from build123d import *

# Parameters (mm, degrees)
SKETCH_1_W          = 275.5
SKETCH_1_H          = 88.9
EXTRUDE_1_DEPTH     = 10
FILLET_1_R          = 10
CUT_EXTRUDE_1_DEPTH = 10
CHAMFER_2_SIZE      = 2
FILLET_3_R          = 3
SKETCH_3_W          = 255.5
SKETCH_3_H          = 3
CUT_EXTRUDE_2_DEPTH = 4
SKETCH_4_R          = 1.5
CUT_EXTRUDE_3_DEPTH = 46
CUT_EXTRUDE_START   = -4
SKETCH_5_R          = 3
SKETCH_5_R_2        = 1.5
CUT_EXTRUDE_4_DEPTH = 4
SKETCH_6_W          = 135.5
SKETCH_6_H          = 3
EXTRUDE_2_DEPTH     = 3


with BuildPart() as part:
    # 草图1 → 凸台-拉伸1 (new body)
    with BuildSketch(Plane.XY):
        Rectangle(SKETCH_1_W, SKETCH_1_H)
    extrude(amount=EXTRUDE_1_DEPTH)

    # 圆角1
    fillet_1_edges = [part.edges().sort_by_distance(p)[0] for p in [
        (137.75, -44.45, 5),
        (-137.75, -44.45, 5),
        (-137.75, 44.45, 5),
        (137.75, 44.45, 5),
    ]]
    fillet(fillet_1_edges, radius=FILLET_1_R)

    # 草图2 → 切除-拉伸1 (cut)
    with BuildSketch(Plane.XY.offset(10)):
        with BuildLine():
            Line((-6.25, 30.95), (6.25, 30.95))
            ThreePointArc((6.25, 30.95), (13.321067812, 28.021067812), (16.25, 20.95))
            Line((16.25, 20.95), (16.25, -20.95))
            ThreePointArc((16.25, -20.95), (13.321067812, -28.021067812), (6.25, -30.95))
            Line((6.25, -30.95), (-6.25, -30.95))
            ThreePointArc((-6.25, -30.95), (-13.787950414, -27.521096069), (-16.156519268, -19.58586071))
            Line((-16.156519268, -19.58586071), (-16.156519268, 19.58586071))
            ThreePointArc((-16.156519268, 19.58586071), (-13.787950414, 27.521096069), (-6.25, 30.95))
        make_face()
        with BuildLine():
            Line((-43.75, -30.95), (-56.25, -30.95))
            ThreePointArc((-56.25, -30.95), (-63.787950414, -27.521096069), (-66.156519268, -19.58586071))
            Line((-66.156519268, -19.58586071), (-66.156519268, 19.58586071))
            ThreePointArc((-66.156519268, 19.58586071), (-63.787950414, 27.521096069), (-56.25, 30.95))
            Line((-56.25, 30.95), (-43.75, 30.95))
            ThreePointArc((-43.75, 30.95), (-36.678932188, 28.021067812), (-33.75, 20.95))
            Line((-33.75, 20.95), (-33.75, -20.95))
            ThreePointArc((-33.75, -20.95), (-36.678932188, -28.021067812), (-43.75, -30.95))
        make_face()
        with BuildLine():
            Line((56.25, -30.95), (43.75, -30.95))
            ThreePointArc((43.75, -30.95), (36.212049586, -27.521096069), (33.843480732, -19.58586071))
            Line((33.843480732, -19.58586071), (33.843480732, 19.58586071))
            ThreePointArc((33.843480732, 19.58586071), (36.212049586, 27.521096069), (43.75, 30.95))
            Line((43.75, 30.95), (56.25, 30.95))
            ThreePointArc((56.25, 30.95), (63.321067812, 28.021067812), (66.25, 20.95))
            Line((66.25, 20.95), (66.25, -20.95))
            ThreePointArc((66.25, -20.95), (63.321067812, -28.021067812), (56.25, -30.95))
        make_face()
        with BuildLine():
            Line((106.25, -30.95), (93.75, -30.95))
            ThreePointArc((93.75, -30.95), (86.212049586, -27.521096069), (83.843480732, -19.58586071))
            Line((83.843480732, -19.58586071), (83.843480732, 19.58586071))
            ThreePointArc((83.843480732, 19.58586071), (86.212049586, 27.521096069), (93.75, 30.95))
            Line((93.75, 30.95), (106.25, 30.95))
            ThreePointArc((106.25, 30.95), (113.321067812, 28.021067812), (116.25, 20.95))
            Line((116.25, 20.95), (116.25, -20.95))
            ThreePointArc((116.25, -20.95), (113.321067812, -28.021067812), (106.25, -30.95))
        make_face()
        with BuildLine():
            Line((-93.75, -30.95), (-106.25, -30.95))
            ThreePointArc((-106.25, -30.95), (-113.787950414, -27.521096069), (-116.156519268, -19.58586071))
            Line((-116.156519268, -19.58586071), (-116.156519268, 19.58586071))
            ThreePointArc((-116.156519268, 19.58586071), (-113.787950414, 27.521096069), (-106.25, 30.95))
            Line((-106.25, 30.95), (-93.75, 30.95))
            ThreePointArc((-93.75, 30.95), (-86.678932188, 28.021067812), (-83.75, 20.95))
            Line((-83.75, 20.95), (-83.75, -20.95))
            ThreePointArc((-83.75, -20.95), (-86.678932188, -28.021067812), (-93.75, -30.95))
        make_face()
    extrude(amount=-CUT_EXTRUDE_1_DEPTH, mode=Mode.SUBTRACT)

    # 倒角2
    chamfer_2_edges = [part.edges().sort_by_distance(p)[0] for p in [
        (86.212049586, 27.521096069, 10),
        (83.843480732, 0, 10),
        (86.212049586, -27.521096069, 10),
        (100, -30.95, 10),
        (113.321067812, -28.021067812, 10),
        (116.25, 0, 10),
        (113.321067812, 28.021067812, 10),
        (100, 30.95, 10),
        (-113.787950414, 27.521096069, 10),
        (-116.156519268, 0, 10),
        (-113.787950414, -27.521096069, 10),
        (-100, -30.95, 10),
        (-86.678932188, -28.021067812, 10),
        (-83.75, 0, 10),
        (-86.678932188, 28.021067812, 10),
        (-100, 30.95, 10),
        (-13.787950414, 27.521096069, 10),
        (-16.156519268, 0, 10),
        (-13.787950414, -27.521096069, 10),
        (0, -30.95, 10),
        (13.321067812, -28.021067812, 10),
        (16.25, 0, 10),
        (13.321067812, 28.021067812, 10),
        (0, 30.95, 10),
        (36.212049586, 27.521096069, 10),
        (33.843480732, 0, 10),
        (36.212049586, -27.521096069, 10),
        (50, -30.95, 10),
        (63.321067812, -28.021067812, 10),
        (66.25, 0, 10),
        (63.321067812, 28.021067812, 10),
        (50, 30.95, 10),
        (-63.787950414, 27.521096069, 10),
        (-66.156519268, 0, 10),
        (-63.787950414, -27.521096069, 10),
        (-50, -30.95, 10),
        (-36.678932188, -28.021067812, 10),
        (-33.75, 0, 10),
        (-36.678932188, 28.021067812, 10),
        (-50, 30.95, 10),
    ]]
    chamfer(chamfer_2_edges, length=CHAMFER_2_SIZE)

    # 圆角3
    fillet_3_edges = [part.edges().sort_by_distance(p)[0] for p in [
        (0, -44.45, 10),
        (-137.75, 0, 10),
        (137.75, 0, 10),
        (0, 44.45, 10),
        (-134.821067812, 41.521067812, 10),
        (134.821067812, 41.521067812, 10),
        (134.821067812, -41.521067812, 10),
        (-134.821067812, -41.521067812, 10),
    ]]
    fillet(fillet_3_edges, radius=FILLET_3_R)

    # 草图3 → 切除-拉伸2 (cut)
    with BuildSketch(Plane(origin=(0, 0, 0), x_dir=(-1, 0, 0), z_dir=(0, 0, -1))):
        with Locations((0, -40.45)):
            Rectangle(SKETCH_3_W, SKETCH_3_H)
    extrude(amount=-CUT_EXTRUDE_2_DEPTH, mode=Mode.SUBTRACT)

    # 草图4 → 切除-拉伸3 (cut)
    with BuildSketch(Plane(origin=(0, 0, 0), x_dir=(-1, 0, 0), z_dir=(0, 0, -1))):
        with Locations((-130.75, 37.45)):
            Circle(SKETCH_4_R)
        with Locations((130.75, 37.45)):
            Circle(SKETCH_4_R)
        with Locations((130.75, -37.45)):
            Circle(SKETCH_4_R)
        with Locations((-130.75, -37.45)):
            Circle(SKETCH_4_R)
        with Locations((67.75, 37.45)):
            Circle(SKETCH_4_R)
        with Locations((-130.75, 0)):
            Circle(SKETCH_4_R)
        with Locations((130.75, 0)):
            Circle(SKETCH_4_R)
    extrude(amount=-CUT_EXTRUDE_3_DEPTH, mode=Mode.SUBTRACT)

    # 草图5 → 切除-拉伸4 (cut)
    # profile 1 of 7: a face of its own
    with BuildSketch(Plane.XY.offset(10).offset(CUT_EXTRUDE_START)):
        with Locations((-67.75, 37.45)):
            Circle(SKETCH_5_R)
        with Locations(Location((-67.75, 37.45, 0), (0, 0, 180))):
            Circle(SKETCH_5_R_2, mode=Mode.SUBTRACT)
    # profile 2 of 7: a face of its own
    with BuildSketch(Plane.XY.offset(10).offset(CUT_EXTRUDE_START)):
        with Locations((130.75, 0)):
            Circle(SKETCH_5_R)
        with Locations(Location((130.75, 0, 0), (0, 0, 180))):
            Circle(SKETCH_5_R_2, mode=Mode.SUBTRACT)
    # profile 3 of 7: a face of its own
    with BuildSketch(Plane.XY.offset(10).offset(CUT_EXTRUDE_START)):
        with Locations((-130.75, 0)):
            Circle(SKETCH_5_R)
        with Locations(Location((-130.75, 0, 0), (0, 0, 180))):
            Circle(SKETCH_5_R_2, mode=Mode.SUBTRACT)
    # profile 4 of 7: a face of its own
    with BuildSketch(Plane.XY.offset(10).offset(CUT_EXTRUDE_START)):
        with Locations((-130.75, 37.45)):
            Circle(SKETCH_5_R)
        with Locations(Location((-130.75, 37.45, 0), (0, 0, 180))):
            Circle(SKETCH_5_R_2, mode=Mode.SUBTRACT)
    # profile 5 of 7: a face of its own
    with BuildSketch(Plane.XY.offset(10).offset(CUT_EXTRUDE_START)):
        with Locations((-130.75, -37.45)):
            Circle(SKETCH_5_R)
        with Locations(Location((-130.75, -37.45, 0), (0, 0, 180))):
            Circle(SKETCH_5_R_2, mode=Mode.SUBTRACT)
    # profile 6 of 7: a face of its own
    with BuildSketch(Plane.XY.offset(10).offset(CUT_EXTRUDE_START)):
        with Locations((130.75, 37.45)):
            Circle(SKETCH_5_R)
        with Locations(Location((130.75, 37.45, 0), (0, 0, 180))):
            Circle(SKETCH_5_R_2, mode=Mode.SUBTRACT)
    # profile 7 of 7: a face of its own
    with BuildSketch(Plane.XY.offset(10).offset(CUT_EXTRUDE_START)):
        with Locations((130.75, -37.45)):
            Circle(SKETCH_5_R)
        with Locations(Location((130.75, -37.45, 0), (0, 0, 180))):
            Circle(SKETCH_5_R_2, mode=Mode.SUBTRACT)
    extrude(amount=CUT_EXTRUDE_4_DEPTH, mode=Mode.SUBTRACT)

    # 草图6 → 凸台-拉伸2 (add)
    with BuildSketch(Plane(origin=(0, 0, 0), x_dir=(-1, 0, 0), z_dir=(0, 0, -1))):
        with Locations((-10, 39.45)):
            Rectangle(SKETCH_6_W, SKETCH_6_H)
    extrude(amount=EXTRUDE_2_DEPTH)


solid = part.part
Geometry check sheet. Reference: the model listing, model coordinates, mm. A direction names the side the tool comes from. Round coordinates to 2 decimals unless told otherwise and drop trailing zeros. Order: outer loops, then holes, each group sorted by start corner. A loop starts at its lowest first (then second) coordinate and runs counter-clockwise, first axis right, second up. Notation, with made-up numbers: M 44,18 L 91,18 A33 ccw 91,46 Z; hole C 71.5,-28 d2. An arc over 180 degrees is marked long. Write each question's results on one line, items separated by ' | '. Start each with the question number.
1. Material ranges on L1, parallel to Y at x = 1.5, z = 2.25; L2, parallel to X at y = -4, z = 2.75; L3, parallel to Y at x = 130.75, z = 4.7, recorded low to high. Write a range as from..to.
2. Cross-section at A-A on x = -51. Record the boundary of the cut face in (y, z), plus the area to 3 significant figures.
3. Draft check along Y on faces 1 (the face through (13.786, -28.322, 8.542)), 2 (the face through (86.05, -27.82, 8.32)), 3 (the face through (134.74, -41.6, 3.55)). Enter one of: pulls with the +Y half, pulls with the -Y half, needs draft (parallel to the pull), parting line crosses it, or undercut.
4. Set-up check for faces 4 (the face through (-113.95, -27.82, 8.32)), 5 (the face through (-50, 30.95, 4)), 6 (the face through (-2, -44.45, 3)): record each of +Z, -Z, +X, -X, +Y, -Y from which the full face is reachable in a straight line by a thin tool's end or side.
5. Go/stop test with flat-tipped pins: P1, Ø1, axis at x = 98.5, y = -30.5, coming from the +Z side; P2, Ø1.5, axis at x = 18, y = 34, coming from the -Z side; P3, Ø1.8, axis at x = 131, y = -0.5, coming from the +Z side. Record where each tip stops, or that it passes through.
6. Cross-section at B-B on y = 11. Give the number of separate pieces and of enclosed holes in the cut face, plus the area to 3 significant figures.
Resolved:
1) L1: -44.45..-41.95, -38.95..-30.95, 30.95..44.45 | L2: -137.75..-116.16, -83.75..-66.16, -33.75..-16.16, 16.25..33.84, 66.25..83.84, 116.25..137.75 | L3: -43.99..-38.95, -35.95..-1.5, 1.5..35.95, 38.95..43.99
2) outline: M -44.45,0 L -41.95,0 L -41.95,4 L -38.95,4 L -38.95,0 L -30.95,0 L -30.95,8 L -32.95,10 L -41.45,10 A3 ccw -44.45,7 Z; M 30.95,0 L 37.95,0 L 37.95,-3 L 40.95,-3 L 40.95,0 L 44.45,0 L 44.45,7 A3 ccw 41.45,10 L 32.95,10 L 30.95,8 Z | area: 259 mm2
3) face 1: undercut | face 2: undercut | face 3: pulls with the -Y half
4) face 4: +Z | face 5: +Z, -Z | face 6: +Z, -Z, +X, -X, -Y
5) P1: z = 8.05 | P2: z = 0 | P3: through
6) separate pieces: 6 | enclosed holes: 0 | area: 1,110 mm2
